Geometry check sheet. Reference: the model listing, model coordinates, mm. Coordinates: 2 decimals unless noted, no trailing zeros. Loops run counter-clockwise (first coordinate to the right, second up) from the corner with the lowest first, then second, coordinate; pieces in that order, holes last.
from build123d import *

# Parameters (mm, degrees)
F0_R     = 127
F0_R_2   = 63.5
F1_DEPTH = 20
F2_R     = 5
F3_SIZE  = 5
F4_SIZE  = 5
F5_R     = 5


with BuildPart() as f1:
    # F0 (on Top) → F1 (new body)
    with BuildSketch(Plane.XY):
        Circle(F0_R)
        Circle(F0_R_2, mode=Mode.SUBTRACT)
    extrude(amount=F1_DEPTH)

    # F2
    f2_edges = [f1.edges().sort_by_distance(p)[0] for p in [
        (-63.5, 0, 20),
    ]]
    fillet(f2_edges, radius=F2_R)

    # F3
    f3_edges = [f1.edges().sort_by_distance(p)[0] for p in [
        (-127, 0, 20),
    ]]
    chamfer(f3_edges, length=F3_SIZE)

    # F4
    f4_edges = [f1.edges().sort_by_distance(p)[0] for p in [
        (-127, 0, 0),
    ]]
    chamfer(f4_edges, length=F4_SIZE)

    # F5
    f5_edges = [f1.edges().sort_by_distance(p)[0] for p in [
        (-63.5, 0, 0),
    ]]
    fillet(f5_edges, radius=F5_R)


solid = f1.part
(1) Sectioned sample at C-C on z = 8.75. Record the cut outline in (x, y).
Findings:
outline: circle Ø254 at (0, 0); hole circle Ø127 at (0, 0)
(2) Sectioned sample at A-A on y = 0. Record the cut outline in (x, z), and give its area (3 significant figures).
Findings:
outline: (-127, 5) - (-122, 0) - (-68.5, 0) arc R5 ccw to (-63.5, 5) - (-63.5, 15) arc R5 ccw to (-68.5, 20) - (-122, 20) - (-127, 15) - close; (63.5, 5) arc R5 ccw to (68.5, 0) - (122, 0) - (127, 5) - (127, 15) - (122, 20) - (68.5, 20) arc R5 ccw to (63.5, 15) - close
area: 2,470 mm2
(3) Scan lines: L1, parallel to Y at x = 0, z = 7.25; L2, parallel to Y at x = -12.5, z = 14.5; L3, parallel to X at y = 33, z = 15.75. Record each from-to range of solid material in increasing order.
Findings:
L1: y = -127 to -63.5, 63.5 to 127
L2: y = -126.38 to -62.26, 62.26 to 126.38
L3: x = -121.86 to -54.32, 54.32 to 121.86
(4) Draft check along X on faces 1 (the conical face through (-26.52, -119.4, 19.69)), 2 (the cylindrical face through (-13.77, -61.99, 9.93)), 3 (the flat face through (53, -53, 0)). Enter one of: +X half, -X half, draft (parallel to the pull), parting line (faces both ways), or undercut.
Findings:
face 1: parting line
face 2: undercut
face 3: draft
(5) Gauge pin test, flat ends, axial feed: pin 1 Ø1 at (y, z) = (4.5, 7) entering from +X; pin 2 Ø1 at (y, z) = (-36.5, 13.5) entering from +X; pin 3 Ø10 at (y, z) = (33, 7) entering from -X. Record the tip position at first contact, or that the pin passes through.
Findings:
pin 1: stops at x = 126.94
pin 2: stops at x = 121.79
pin 3: stops at x = -123.87
